The listing builds one solid part. Answer for the finished solid, in the listing's coordinates (mm). Face numbers are marked on the shaded views. Round coordinates to 2 decimals unless told otherwise and drop trailing zeros. Loops run counter-clockwise (first coordinate to the right, second up) from the corner with the lowest first, then second, coordinate; pieces in that order, holes last. Notation, with made-up numbers: (32.25, -21.75) - (42.25, -21.75) arc R10 cw to (42.25, -4.75) - close; hole circle Ø8 at (36, -27.5). An arc over 180 degrees is marked (long way). Write item = value, one per line. Start each with the question number.
1) Section C-C, the plane z = 62 is taken. Determine the outline of the cut face in (x, y), and give its area (3 significant figures).
2) Given pin 1 Ø8 at (x, y) = (24, 12) entering from +Z; pin 2 Ø9 at (x, z) = (-39.96, 25.03) entering from -Y; pin 3 Ø1.5 at (x, y) = (-26, 5) entering from -Z; pin 4 Ø1.5 at (x, y) = (15, 13) entering from +Z, each flat-ended and moving along its own axis, determine where each tip first touches the part or whether it passes through.
3) For a pull along Z with two mould halves and no side action, classify the marked faces 1 and 2 as released by +Z, released by -Z, zero draft, split by the parting line, or undercut.
4) Straight lines are drawn through the part: line 1 along Z through (x, y) = (0, 0.5); line 2 along Y through (x, z) = (-44, 55); line 3 along Z through (x, y) = (-44.5, -1). For each, find the intervals that lie inside material, in ascending order.
5) Section D-D, the plane x = 60 is taken. Determine the outline of the cut face in (y, z), and give its area (3 significant figures).
6) Section B-B, the plane z = 0 is taken. Give the number of separate pieces and of enclosed holes in the cut face, and give its area (3 significant figures).
from build123d import *

# Parameters (mm, degrees)
SKETCH6_R                                = 66.04
BOSS_EXTRUDE1_DEPTH                      = 2.54
PIPE_TAP_DRILL_FOR_1_4_TAP_GN2_D         = 11.1252
SKETCH7_R                                = 6.35
CUT_EXTRUDE1_SIPHON_DEPTH                = 105.994177492
PIPE_TAP_DRILL_FOR_1_4_TAP_RELIEF_VALV_D = 11.1252
PIPE_TAP_DRILL_FOR_1_4_TAP_VENT_VALVE_D  = 11.1252


with BuildPart() as part:
    # Sketch1 → Revolve1 (revolve)
    with BuildSketch(Plane.XY, mode=Mode.PRIVATE) as revolve1_sk:
        Polygon((0, 0), (72.898, 0), (72.898, 2.4638), (69.977, 2.4638), (69.977, 7.4422), (72.898, 7.4422), (72.898, 9.906), (69.977, 9.906), (69.977, 14.986), (72.898, 14.986), (72.898, 17.3482), (66.548, 17.3482), (66.548, 6.35), (0, 6.35), align=None)
    revolve(revolve1_sk.sketch.rotate(Axis((0, 48.192213231, 0), (0, -1, 0)), 180), axis=Axis((0, 48.192213231, 0), (0, -1, 0)))

    # Sketch6 → Boss-Extrude1 (add)
    with BuildSketch(Plane.XZ):
        Circle(SKETCH6_R)
    extrude(amount=BOSS_EXTRUDE1_DEPTH)

    # Pipe Tap Drill for 1/4 Tap - GN2 (through all)
    with Locations(Plane(origin=(0, 6.35, 0), x_dir=(1, 0, 0), z_dir=(0, 1, 0))):
        with Locations((0, 0)):
            Hole(PIPE_TAP_DRILL_FOR_1_4_TAP_GN2_D / 2)

    # Sketch7 → Cut-Extrude1-Siphon (cut, through all)
    with BuildSketch(Plane(origin=(0, -2.54, 0), x_dir=(-1, 0, 0), z_dir=(0, -1, 0))):
        with Locations(Location((-38.1, 0, 0), (0, 0, 180))):
            Circle(SKETCH7_R)
    extrude(amount=-CUT_EXTRUDE1_SIPHON_DEPTH, mode=Mode.SUBTRACT)

    # Pipe Tap Drill for 1/4 Tap - Relief Valve (through all)
    with Locations(Plane(origin=(0, -2.54, 0), x_dir=(-1, 0, 0), z_dir=(0, -1, 0))):
        with Locations((40.358041229, 19.878625199)):
            Hole(PIPE_TAP_DRILL_FOR_1_4_TAP_RELIEF_VALV_D / 2)

    # Pipe Tap Drill for 1/4 Tap - Vent Valve (through all)
    with Locations(Plane(origin=(0, -2.54, 0), x_dir=(-1, 0, 0), z_dir=(0, -1, 0))):
        with Locations((39.961427255, -25.031151171)):
            Hole(PIPE_TAP_DRILL_FOR_1_4_TAP_VENT_VALVE_D / 2)


solid = part.part
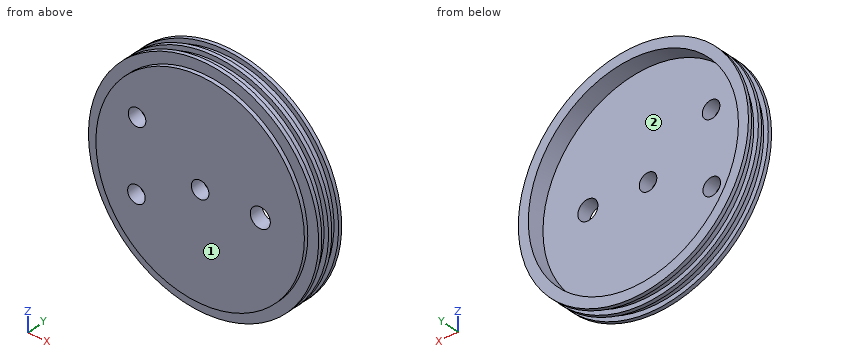
Geometry check:
q1.outline = (-38.34, 0) - (-22.74, 0) - (-22.74, -2.54) - (22.74, -2.54) - (22.74, 0) - (38.34, 0) - (38.34, 2.46) - (32.45, 2.46) - (32.45, 7.44) - (38.34, 7.44) - (38.34, 9.91) - (32.45, 9.91) - (32.45, 14.99) - (38.34, 14.99) - (38.34, 17.35) - (24.18, 17.35) - (24.18, 6.35) - (-24.18, 6.35) - (-24.18, 17.35) - (-38.34, 17.35) - (-38.34, 14.99) - (-32.45, 14.99) - (-32.45, 9.91) - (-38.34, 9.91) - (-38.34, 7.44) - (-32.45, 7.44) - (-32.45, 2.46) - (-38.34, 2.46) - close
q1.area = 795 mm2
q2.pin_1 = 69.93
q2.pin_2 = through
q2.pin_3 = -65.26
q2.pin_4 = 68.51
q3.face_1 = zero draft
q3.face_2 = undercut
q4.line_1 = -72.9 to -5.56, 5.56 to 72.9
q4.line_2 = 0 to 2.46, 7.44 to 9.91, 14.99 to 17.35
q4.line_3 = -48.8 to -23.59, -16.17 to 21.81, 28.25 to 48.8
q5.outline = (-2.54, -27.59) - (0, -27.59) - (0, -41.4) - (2.46, -41.4) - (2.46, -36.01) - (7.44, -36.01) - (7.44, -41.4) - (9.91, -41.4) - (9.91, -36.01) - (14.99, -36.01) - (14.99, -41.4) - (17.35, -41.4) - (17.35, -28.79) - (6.35, -28.79) - (6.35, 28.79) - (17.35, 28.79) - (17.35, 41.4) - (14.99, 41.4) - (14.99, 36.01) - (9.91, 36.01) - (9.91, 41.4) - (7.44, 41.4) - (7.44, 36.01) - (2.46, 36.01) - (2.46, 41.4) - (0, 41.4) - (0, 27.59) - (-2.54, 27.59) - close
q5.area = 835 mm2
q6.separate_pieces = 3
q6.enclosed_holes = 0
q6.area = 1,130 mm2
